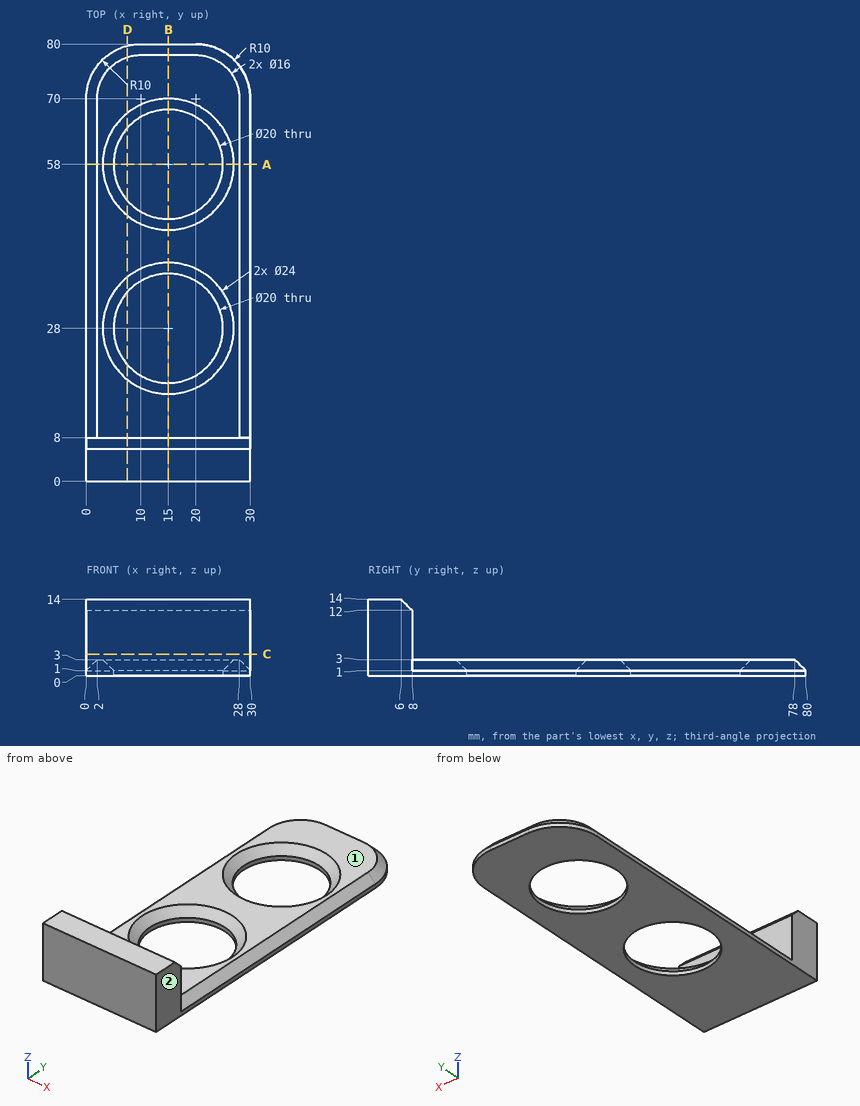
Here's the drawing with two shaded views (mm, measured from the low corner). I have some questions. A direction names the side the tool comes from. Give positions to 0.01 mm unless a question says otherwise; leave off trailing zeros. Order: outer loops, then holes, each group sorted by start corner. A loop starts at its lowest first (then second) coordinate and runs counter-clockwise, first axis right, second up. Notation, with made-up numbers: (-13.5, -20.5) - (28.5, -20.5) arc R19 ccw to (28.5, 7.5) - close; hole circle Ø3 at (29.25, 70.5). An arc over 180 degrees is marked (long way). Use a Markdown table: item, result. Add a question column.
Q1. If we section it at D-D on x = 7.5: Count the separate pieces of the cut face and the enclosed holes in it, plus the area to 3 significant figures.
Q2. If we section it at B-B on x = 15: Write out the boundary of the cut face in (y, z), plus the area to 3 significant figures.
Q3. Please list where these lines run through material, in increasing order: line 1 along Y through (x, z) = (15, 0.6); line 2 along Y through (x, z) = (28.5, 8.5); line 3 along Z through (x, y) = (24, 10).
Q4. If we section it at C-C on z = 4: Write out the boundary of the cut face in (x, y).
Q5. I'm going to push flat-ended pins straight in: pin 1 (12 mm diameter, centred on x = 15, y = 28, fed in from -Z); pin 2 (5.5 mm diameter, centred on x = 19, z = 5, fed in from +Y); pin 3 (2 mm diameter, centred on x = 6, y = 44, fed in from +Z); pin 4 (4 mm diameter, centred on x = 8, z = 6.5, fed in from +Y). Where does each tip first touch, or does it pass through?
Q6. If we section it at A-A on y = 58: Write out the boundary of the cut face in (x, z), plus the area to 3 significant figures.
Q7. On a 3-axis mill with a long thin cutter (end or side, diameter ignored), from which of +Z, -Z, +X, -X, +Y, -Y can I reach the whole of each face in a straight line? I mean the marked faces 1 and 2. Say none if no direction works.
Answers follow:
| question | item | result |
|---|---|---|
| 1 | separate pieces | 3 |
| 1 | enclosed holes | 0 |
| 1 | area | 232 mm^2 |
| 2 | outline | (0, 0) - (18, 0) - (18, 1) - (16, 3) - (8, 3) - (8, 12) - (6, 14) - (0, 14) - close; (38, 0) - (48, 0) - (48, 1) - (46, 3) - (40, 3) - (38, 1) - close; (68, 0) - (80, 0) - (80, 1) - (78, 3) - (70, 3) - (68, 1) - close |
| 2 | area | 196 mm^2 |
| 3 | line 1 | y = 0 to 18, 38 to 48, 68 to 80 |
| 3 | line 2 | y = 0 to 8 |
| 3 | line 3 | z = 0 to 3 |
| 4 | outline | (0, 0) - (30, 0) - (30, 8) - (0, 8) - close |
| 5 | pin 1 | passes through |
| 5 | pin 2 | stops at y = 78.75 |
| 5 | pin 3 | stops at z = 3 |
| 5 | pin 4 | stops at y = 8 |
| 6 | outline | (0, 0) - (5, 0) - (5, 1) - (3, 3) - (2, 3) - (0, 1) - close; (25, 0) - (30, 0) - (30, 1) - (28, 3) - (27, 3) - (25, 1) - close |
| 6 | area | 22.0 mm^2 |
| 7 | face 1 | +Z, +X, -X, +Y |
| 7 | face 2 | +Z, -Z, +X, +Y, -Y |
